```python
from build123d import *

# Parameters (mm, degrees)
SKETCH1_W           = 35
SKETCH1_H           = 20
BOSS_EXTRUDE1_DEPTH = 10
FILLET1_R           = 5
SKETCH4_R           = 6
CUT_EXTRUDE2_DEPTH  = 23.5
SKETCH5_W           = 4.5
SKETCH5_H           = 20
BOSS_EXTRUDE3_DEPTH = 28
SKETCH6_R           = 1.85
CUT_EXTRUDE3_DEPTH  = 43.594013664


with BuildPart() as part:
    # Sketch1 → Boss-Extrude1 (new body)
    with BuildSketch(Plane(origin=(0, 0, 0), x_dir=(1, 0, 0), z_dir=(0, 1, 0))):
        Rectangle(SKETCH1_W, SKETCH1_H)
    extrude(amount=BOSS_EXTRUDE1_DEPTH)

    # Fillet1
    fillet1_edges = [part.edges().sort_by_distance(p)[0] for p in [
        (17.5, 5, 10),
        (17.5, 5, -10),
    ]]
    fillet(fillet1_edges, radius=FILLET1_R)

    # Sketch4 → Cut-Extrude2 (cut, through all)
    with BuildSketch(Plane(origin=(0, 10, 0), x_dir=(1, 0, 0), z_dir=(0, 1, 0))):
        with Locations(Location((6.5, 0, 0), (0, 0, 270))):
            Circle(SKETCH4_R)
    extrude(amount=-CUT_EXTRUDE2_DEPTH, mode=Mode.SUBTRACT)

    # Sketch5 → Boss-Extrude3 (add)
    with BuildSketch(Plane.XZ):
        with Locations((-15.25, 0)):
            Rectangle(SKETCH5_W, SKETCH5_H)
    extrude(amount=BOSS_EXTRUDE3_DEPTH)

    # Sketch6 → Cut-Extrude3 (cut, through all)
    with BuildSketch(Plane(origin=(-13, 0, 0), x_dir=(0, 0, -1), z_dir=(1, 0, 0))):
        with Locations((0, -6)):
            Circle(SKETCH6_R)
        with Locations((0, -21)):
            Circle(SKETCH6_R)
    extrude(amount=-CUT_EXTRUDE3_DEPTH, mode=Mode.SUBTRACT)


solid = part.part
```
CAD build for the part. Positions are in the model's coordinates, mm. A direction names the side the tool comes from. Give positions to 0.01 mm unless a question says otherwise; leave off trailing zeros. Write each loop counter-clockwise with the first axis right and the second up, starting at its lowest first coordinate (ties: lowest second). Pieces come first, ordered by that corner, then holes. Notation, with made-up numbers: M 54.5,30 L 113.5,30 A20 cw 113.5,34 Z; hole C 2,-35.5 d9. An arc over 180 degrees is marked long. Return JSON: item names as keys, results as strings. Group by question number.
(1) Band-saw the part on C-C (z = 0). Give the cut face in (x, y), and give its area (3 significant figures).
(2) Band-saw the part on D-D (y = 5). Give the cut face in (x, z), and give its area (3 significant figures).
(3) Flat gauge pins, fed straight in: pin 1 Ø10 at (x, z) = (7, 6) entering from -Y; pin 2 Ø4.5 at (y, z) = (-6, 0) entering from +X. Where does each tip first touch, or does it go through?
(4) Band-saw the part on A-A (x = 6.5). Give the cut face in (y, z).
(5) Mould opens along Z. For faces 1 (the face through (-6, 1, -10)), 2 (the face through (-17.5, -9, 0)), 3 (the face through (-6, 1, 10)), 4 (the face through (-15.218, -19.166, 0.241)) say: pulls with the +Z half, pulls with the -Z half, needs draft (parallel to the pull), parting line crosses it, or undercut.
(6) Band-saw the part on B-B (y = -21). Give the cut face in (x, z).
(7) Drill centre lines: L1, parallel to Y at x = -15.95, z = 0; L2, parallel to X at y = 7, z = 0; L3, parallel to X at y = -24, z = -1. Where is each one in solid material? Low to high. Write a range as [from, to].
(8) 3-axis set-ups, long thin cutter, end or side, ignore diameter. For faces 5 (the face through (-15, -28, 0)), 6 (the face through (-1, 0, 0)): which of +Z, -Z, +X, -X, +Y, -Y reach the whole face in a straight line?
Entries:
{
 "1": {"outline": "M -17.5,-28 L -13,-28 L -13,-22.85 L -17.5,-22.85 Z; M -17.5,-19.15 L -13,-19.15 L -13,-7.85 L -17.5,-7.85 Z; M -17.5,-4.15 L -13,-4.15 L -13,0 L 0.5,0 L 0.5,10 L -17.5,10 Z; M 12.5,0 L 17.5,0 L 17.5,10 L 12.5,10 Z", "area": "323 mm^2"},
 "2": {"outline": "M -17.5,-10 L 12.5,-10 A5 ccw 17.5,-5 L 17.5,5 A5 ccw 12.5,10 L -17.5,10 Z; hole C 6.5,0 d12", "area": "576 mm^2"},
 "3": {"pin 1": "stops at y = 0", "pin 2": "stops at x = -13"},
 "4": {"outline": "M 0,-10 L 10,-10 L 10,-6 L 0,-6 Z; M 0,6 L 10,6 L 10,10 L 0,10 Z"},
 "5": {"face 1": "pulls with the -Z half", "face 2": "needs draft", "face 3": "pulls with the +Z half", "face 4": "undercut"},
 "6": {"outline": "M -17.5,-10 L -13,-10 L -13,-1.85 L -17.5,-1.85 Z; M -17.5,1.85 L -13,1.85 L -13,10 L -17.5,10 Z"},
 "7": {"L1": "y = [-28, -22.85], [-19.15, -7.85], [-4.15, 10]", "L2": "x = [-17.5, 0.5], [12.5, 17.5]", "L3": "x = [-17.5, -13]"},
 "8": {"face 5": "+Z, -Z, +X, -X, -Y", "face 6": "+Z, -Z, +X, -Y"}
}
